The model under review builds one solid part; all positions refer to its coordinate system, in mm. Round coordinates to 2 decimals unless told otherwise and drop trailing zeros. Loops run counter-clockwise (first coordinate to the right, second up) from the corner with the lowest first, then second, coordinate; pieces in that order, holes last. Notation, with made-up numbers: M 71.5,37 L 97.5,37 A8 ccw 97.5,45 Z; hole C -40,29 d6. An arc over 180 degrees is marked long. Use a Markdown table: item, result. Add a question column.
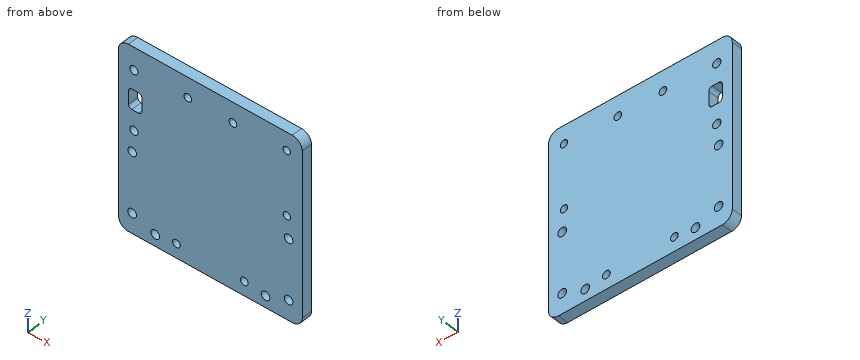
```python
from build123d import *

# Parameters (mm, degrees)
SKETCH1_W           = 55
SKETCH1_H           = 55
BOSS_EXTRUDE1_DEPTH = 3.175
SKETCH2_R           = 1.3
CUT_EXTRUDE1_DEPTH  = 3.175
FILLET1_R           = 3
SKETCH3_R           = 1.25
SKETCH3_R_2         = 1.1
CUT_EXTRUDE2_DEPTH  = 3.175
SKETCH4_R           = 1.15
CUT_EXTRUDE3_DEPTH  = 3.175
SKETCH5_R           = 1.15
CUT_EXTRUDE4_DEPTH  = 3.175
SKETCH6_R           = 1.3
CUT_EXTRUDE5_DEPTH  = 3.175
CUT_EXTRUDE6_DEPTH  = 3.175


with BuildPart() as part:
    # Sketch1 → Boss-Extrude1 (new body)
    with BuildSketch(Plane(origin=(0, 0, 0), x_dir=(1, 0, 0), z_dir=(0, 1, 0))):
        Rectangle(SKETCH1_W, SKETCH1_H)
    extrude(amount=BOSS_EXTRUDE1_DEPTH)

    # Sketch2 → Cut-Extrude1 (cut)
    with BuildSketch(Plane(origin=(0, 3.175, 0), x_dir=(1, 0, 0), z_dir=(0, 1, 0))):
        with Locations((-23.4, 21.5)):
            Circle(SKETCH2_R)
        with Locations((-23.4, 3.5)):
            Circle(SKETCH2_R)
        with Locations((23.4, 3.5)):
            Circle(SKETCH2_R)
        with Locations((23.4, 21.5)):
            Circle(SKETCH2_R)
    extrude(amount=-CUT_EXTRUDE1_DEPTH, mode=Mode.SUBTRACT)

    # Fillet1
    fillet1_edges = [part.edges().sort_by_distance(p)[0] for p in [
        (27.5, 1.5875, 27.5),
        (-27.5, 1.5875, 27.5),
        (-27.5, 1.5875, -27.5),
        (27.5, 1.5875, -27.5),
    ]]
    fillet(fillet1_edges, radius=FILLET1_R)

    # Sketch3 → Cut-Extrude2 (cut)
    with BuildSketch(Plane(origin=(0, 3.175, 0), x_dir=(1, 0, 0), z_dir=(0, 1, 0))):
        with Locations((-22.865, -3)):
            Circle(SKETCH3_R)
        with Locations((22.855, -3)):
            Circle(SKETCH3_R_2)
        with Locations((22.855, -22.11)):
            Circle(SKETCH3_R_2)
        with Locations((-22.865, -20.78)):
            Circle(SKETCH3_R)
    extrude(amount=-CUT_EXTRUDE2_DEPTH, mode=Mode.SUBTRACT)

    # Sketch4 → Cut-Extrude3 (cut)
    with BuildSketch(Plane(origin=(0, 3.175, 0), x_dir=(1, 0, 0), z_dir=(0, 1, 0))):
        with Locations((-10.16, 23.24)):
            Circle(SKETCH4_R)
        with Locations((10.16, 23.24)):
            Circle(SKETCH4_R)
    extrude(amount=-CUT_EXTRUDE3_DEPTH, mode=Mode.SUBTRACT)

    # Sketch5 → Cut-Extrude4 (cut)
    with BuildSketch(Plane(origin=(0, 3.175, 0), x_dir=(1, 0, 0), z_dir=(0, 1, 0))):
        with Locations((-6.75, -21.45)):
            Circle(SKETCH5_R)
        with Locations((6.75, -21.45)):
            Circle(SKETCH5_R)
    extrude(amount=-CUT_EXTRUDE4_DEPTH, mode=Mode.SUBTRACT)

    # Sketch6 → Cut-Extrude5 (cut)
    with BuildSketch(Plane(origin=(0, 3.175, 0), x_dir=(1, 0, 0), z_dir=(0, 1, 0))):
        with Locations((-16.5, 24)):
            Circle(SKETCH6_R)
        with Locations((16.5, 24)):
            Circle(SKETCH6_R)
    extrude(amount=-CUT_EXTRUDE5_DEPTH, mode=Mode.SUBTRACT)

    # Sketch7 → Cut-Extrude6 (cut)
    with BuildSketch(Plane(origin=(0, 3.175, 0), x_dir=(1, 0, 0), z_dir=(0, 1, 0))):
        with BuildLine():
            Line((-23.5, -8.89), (-21.5, -8.89))
            ThreePointArc((-21.5, -8.89), (-20.792893219, -9.182893219), (-20.5, -9.89))
            Line((-20.5, -9.89), (-20.5, -13.89))
            ThreePointArc((-20.5, -13.89), (-20.792893219, -14.597106781), (-21.5, -14.89))
            Line((-21.5, -14.89), (-23.5, -14.89))
            ThreePointArc((-23.5, -14.89), (-24.207106781, -14.597106781), (-24.5, -13.89))
            Line((-24.5, -13.89), (-24.5, -9.89))
            ThreePointArc((-24.5, -9.89), (-24.207106781, -9.182893219), (-23.5, -8.89))
        make_face()
    extrude(amount=-CUT_EXTRUDE6_DEPTH, mode=Mode.SUBTRACT)


solid = part.part
```
(1) Insertion check: pin 1 Ø2.5 at (x, z) = (-23.4, -21.5) entering from -Y. The pin has a flat end and moves straight along its axis. Give the tip position at first contact, or say it passes through.
(2) Consider section A-A, the plane x = 16.5. Give the boundary of the cut face in (y, z) (3 decimals).
(3) Consider section C-C, the plane x = -16. Give the boundary of the cut face in (y, z) (3 decimals).
(4) To check wall thickness, follow probe 1 along X at (y, z) = (2.1, 3) (3 decimals); probe 2 along X at (y, z) = (0.95, -21.5); probe 3 along X at (y, z) = (1.45, 10). State the ranges of each line that lie inside material, in increasing order.
(5) Consider section B-B, the plane y = 2.1. Give the number of separate pieces and of enclosed holes in the cut face, then the cut area to 3 significant figures.
Found:
| question | item | result |
|---|---|---|
| 1 | pin 1 | passes through |
| 2 | outline | M 0,-27.5 L 3.175,-27.5 L 3.175,-25.3 L 0,-25.3 Z; M 0,-22.7 L 3.175,-22.7 L 3.175,27.5 L 0,27.5 Z |
| 3 | outline | M 0,-27.5 L 3.175,-27.5 L 3.175,-25.2 L 0,-25.2 Z; M 0,-22.8 L 3.175,-22.8 L 3.175,27.5 L 0,27.5 Z |
| 4 | probe 1 | x = -27.5 to -24.115, -21.615 to 21.755, 23.955 to 27.5 |
| 4 | probe 2 | x = -27.5 to -24.7, -22.1 to 22.1, 24.7 to 27.5 |
| 4 | probe 3 | x = -27.5 to -24.5, -20.5 to 27.5 |
| 5 | separate pieces | 1 |
| 5 | enclosed holes | 15 |
| 5 | area | 2,930 mm^2 |
